```python
from build123d import *

# Parameters (mm, degrees)
IZIM1_R                     = 5
IZIM1_R_2                   = 12.5
Y_KSEKLIK_EKSTR_ZYON1_DEPTH = 5
IZIM2_R                     = 5
KES_EKSTR_ZYON1_DEPTH       = 15
IZIM1_3_R                   = 12.5
Y_KSEKLIK_EKSTR_ZYON2_DEPTH = 143


with BuildPart() as part:
    # Çizim1 → Yükseklik-Ekstrüzyon1 (new, symmetric)
    with BuildSketch(Plane.XY):
        with BuildLine():
            Line((-350, 20), (350, 20))
            ThreePointArc((350, 20), (370, 0), (350, -20))
            Line((350, -20), (-350, -20))
            ThreePointArc((-350, -20), (-370, 0), (-350, 20))
        make_face()
        with Locations((350, 0)):
            Circle(IZIM1_R, mode=Mode.SUBTRACT)
        with Locations((-350, 0)):
            Circle(IZIM1_R_2, mode=Mode.SUBTRACT)
    extrude(amount=Y_KSEKLIK_EKSTR_ZYON1_DEPTH, both=True)

    # Çizim2 → Kes-Ekstrüzyon1 (cut)
    with BuildSketch(Plane.XY.offset(5)):
        Circle(IZIM2_R)
    extrude(amount=-KES_EKSTR_ZYON1_DEPTH, mode=Mode.SUBTRACT)

    # Çizim1<3> → Yükseklik-Ekstrüzyon2 (add)
    with BuildSketch(Plane.XY):
        with Locations((-350, 0)):
            Circle(IZIM1_3_R)
    extrude(amount=Y_KSEKLIK_EKSTR_ZYON2_DEPTH)


solid = part.part
```
The listing builds one solid part. Answer for the finished solid, in the listing's coordinates (mm). A direction names the side the tool comes from. Give positions to 0.01 mm unless a question says otherwise; leave off trailing zeros. Write each loop counter-clockwise with the first axis right and the second up, starting at its lowest first coordinate (ties: lowest second). Pieces come first, ordered by that corner, then holes. Notation, with made-up numbers: (47.5, 51.25) -> (53.5, 51.25) arc R31 ccw to (53.5, 84.25) -> close; hole circle Ø8 at (-38.5, 82). An arc over 180 degrees is marked (long way). Write item = value, one per line. Start each with the question number.
1) Which of the six approach directions +Z, -Z, +X, -X, +Y, -Y give full straight-line access (tool end or side, diameter ignored) to faces 1 (the face through (-338.077, 3.755, -2.535)), 2 (the face through (-370, 0, 0))?
2) The part is cut by section A-A, the plane z = 100.5. Determine the outline of the cut face in (x, y).
3) Determine the mould class of faces 3 (the face through (-338.077, 3.755, 73.034)), 4 (the face through (-350, 0, 0)), 5 (the face through (5.2, 0.3, -5)), 6 (the face through (370, 0, 0)) for opening direction X: +X half, -X half, draft (parallel to the pull), parting line (faces both ways), or undercut.
4) Each of these flat-tipped pins is pushed along its axis until it touches: pin 1 (6 mm diameter, centred on y = 2, z = 58, fed in from +X); pin 2 (12 mm diameter, centred on x = 133, y = 7.5, fed in from +Z); pin 3 (2 mm diameter, centred on y = 1, z = 118, fed in from -X). Where does it stop, or does it pass through?
5) The part is cut by section B-B, the plane x = -195.5. Determine the outline of the cut face in (y, z).
6) Straight lines are drawn through the part: line 1 along Y through (x, z) = (0, -2); line 2 along Y through (x, z) = (-350, -2); line 3 along Z through (x, y) = (-192.5, 5.5). For each, find the intervals that lie inside material, in ascending order.
Solutions:
q1.face_1 = -Z
q1.face_2 = +Z, -Z, -X
q2.outline = circle Ø25 at (-350, 0)
q3.face_3 = parting line
q3.face_4 = undercut
q3.face_5 = draft
q3.face_6 = +X half
q4.pin_1 = -337.5
q4.pin_2 = 5
q4.pin_3 = -362.5
q5.outline = (-20, -5) -> (20, -5) -> (20, 5) -> (-20, 5) -> close
q6.line_1 = -20 to -5, 5 to 20
q6.line_2 = -20 to -12.5, 12.5 to 20
q6.line_3 = -5 to 5
